Can you work these out from the model? Positions are in its coordinate system, mm. A direction names the side the tool comes from. Give positions to 0.01 mm unless a question says otherwise; leave off trailing zeros. Write each loop counter-clockwise with the first axis right and the second up, starting at its lowest first coordinate (ties: lowest second). Pieces come first, ordered by that corner, then holes. Notation, with made-up numbers: (62, 29.25) -> (112, 29.25) arc R17 cw to (112, 35.25) -> close; hole circle Ø10 at (-28, 0). An arc over 180 degrees is marked (long way). One line per item, written item: value.
Autodesk Inventor part; units mm, degrees
ref_plane "YZ Plane" through (0, 0, 0) normal (1, 0, 0) x (0, 1, 0)
ref_plane "XZ Plane" through (0, 0, 0) normal (0, 1, 0) x (-1, 0, 0)
ref_plane "XY Plane" through (0, 0, 0) normal (0, 0, 1) x (1, 0, 0)
sketch "Sketch1" plane through (0, 0, 0) normal (0, 0, 1) x (1, 0, 0)
  line L0 (0, 0) -> (110, 0)
  line L1 (110, 0) -> (110, 65)
  line L2 (110, 65) -> (0, 65)
  line L3 (0, 65) -> (0, 0)
  line L4 (5, 5) -> (105, 5)
  line L5 (105, 5) -> (105, 60)
  line L6 (105, 60) -> (5, 60)
  line L7 (5, 60) -> (5, 5)
  dimension "d0" = 65
  dimension "d1" = 110
  dimension "d4" = 5
extrude "Extrusion1" add sketch "Sketch1" along normal blind 5 contours L3 L2 L1 L0 | L7 L6 L5 L4
extrude "Extrusion2" cut sketch "Sketch1" along normal blind 5 contours L7 L6 L5 L4
sketch "Sketch2" plane through (0, 65, 0) normal (0, 1, 0) x (1, 0, 0)
  line L0 (110, 0) -> (110, -5)
  line L1 (110, 0) -> (0, 0)
  line L2 (0, 0) -> (0, -5)
  point P0 (2.5, -2.5)
  point P1 (107.5, -2.5)
  dimension "d14" = 2.5
  dimension "d15" = 2.5
  dimension "d16" = 2.5
  dimension "d17" = 2.5
hole "Hole1" at (2.5, 65, 2.5) at (107.5, 65, 2.5) direction (0, -1, 0) diameter 2.459 depth 7 tip angle 118
sketch "Sketch4" plane through (5, 5, 0) normal (0, 1, 0) x (1, 0, 0)
  line L0 (0, 0) -> (0, -5) construction
  line L1 (0, -2.5) -> (100, -2.5) construction
  line L2 (100, 0) -> (100, -5) construction
  point P0 (-5, 0)
  point P1 (75, -2.5)
  point P2 (25, -2.5)
  dimension "d36" = 25
  dimension "d37" = 25
hole "Hole3" at (80, 5, 2.5) at (30, 5, 2.5) direction (0, -1, 0) diameter 3 depth 8.8 tip angle 118
properties part number "Camera plate shell" material "Aluminum 6061"
1) For faces 1 (the face through (106.463, 61.451, 3.161)), 2 (the face through (51, 4, 5)), 3 (the face through (28.513, 2.465, 2.305)), 4 (the face through (105, 32, 2)), which set-ups out of +Z, -Z, +X, -X, +Y, -Y let a thin tool reach every point of the face, with its end or its side?
Answer list:
face 1: +Y
face 2: +Z, +X, -X, +Y, -Y
face 3: -Y
face 4: +Z, -Z
2) I need wall thicknesses on L1, parallel to Z at x = 80, y = 1; L2, parallel to Y at x = 95, z = 3.85; L3, parallel to X at y = 41, z = 0.75. Which ranges of each line are inside material? Lowest first, please.
Answer list:
L1: z = 0 to 1, 4 to 5
L2: y = 0 to 5, 60 to 65
L3: x = 0 to 5, 105 to 110
3) We'd pull the mould along X, two halves only. Please class faces 5 (the face through (56, 65, 2)), 6 (the face through (110, 32, 2)), 7 (the face through (78.735, 2.465, 3.306)): released by +X, released by -X, zero draft, split by the parting line, or undercut.
Answer list:
face 5: zero draft
face 6: released by +X
face 7: undercut
4) If we section it at A-A (y = 16.5): Write out the boundary of the cut face in (x, z), and give its area (3 significant figures).
Answer list:
outline: (0, 0) -> (5, 0) -> (5, 5) -> (0, 5) -> close; (105, 0) -> (110, 0) -> (110, 5) -> (105, 5) -> close
area: 50.0 mm^2
5) If we section it at B-B (x = 30): Write out the boundary of the cut face in (y, z).
Answer list:
outline: (0, 0) -> (5, 0) -> (5, 1) -> (0, 1) -> close; (0, 4) -> (5, 4) -> (5, 5) -> (0, 5) -> close; (60, 0) -> (65, 0) -> (65, 5) -> (60, 5) -> close
6) If we section it at C-C (x = 95.5): Write out the boundary of the cut face in (y, z), and give its area (3 significant figures).
Answer list:
outline: (0, 0) -> (5, 0) -> (5, 5) -> (0, 5) -> close; (60, 0) -> (65, 0) -> (65, 5) -> (60, 5) -> close
area: 50.0 mm^2
7) Will these pins go through, and if not, where does the flat tip stop? pin 1 (1.5 mm diameter, centred on x = 107.5, z = 2.5, fed in from +Y); pin 2 (3 mm diameter, centred on y = 35.5, z = 0.5, fed in from -X).
Answer list:
pin 1: stops at y = 57.71
pin 2: stops at x = 0
